Could you check a few things on this model? Use its own coordinates, in mm. A direction names the side the tool comes from. Coordinates: 2 decimals unless noted, no trailing zeros. Loops run counter-clockwise (first coordinate to the right, second up) from the corner with the lowest first, then second, coordinate; pieces in that order, holes last.
1) Imagine slicing it at B-B on z = 3. Please give me the cut outline in (x, y), plus the area to 3 significant figures.
2) If I drill on line 1 along X through (y, z) = (1, 12); line 2 along X through (y, z) = (-1.75, 9.75); line 3 along X through (y, z) = (-0.75, 12), over which ranges is the centre line in solid material (lowest first)?
3) For faces 1 (the face through (0, 0, 0)), 2 (the face through (0, 1.75, 12)), 3 (the face through (0, -2, 5)), which set-ups out of +Z, -Z, +X, -X, +Y, -Y let a thin tool reach every point of the face, with its end or its side?
4) Will these pins go through, and if not, where does the flat tip stop? P1, Ø4, axis at y = 1, z = 6, coming from the -X side; P2, Ø3, axis at x = -1.5, z = 7.5, coming from the +Y side; P3, Ø1, axis at x = -0.5, z = 11.5, coming from the +Y side.
5) Imagine slicing it at A-A on z = 10.75. Please give me the cut outline in (x, y).
```python
from build123d import *

# Parameters (mm, degrees)
SKETCH_1_R          = 2
EXTRUDE_1_DEPTH     = 10
SKETCH_2_R          = 4
EXTRUDE_2_DEPTH     = 3
CUT_EXTRUDE_1_DEPTH = 2
FILLET_1_R          = 2


with BuildPart() as part:
    # 草图1 → 凸台-拉伸1 (new body)
    with BuildSketch(Plane.XY):
        Circle(SKETCH_1_R)
    extrude(amount=EXTRUDE_1_DEPTH)

    # 草图2 → 凸台-拉伸2 (add)
    with BuildSketch(Plane.XY.offset(10)):
        Circle(SKETCH_2_R)
    extrude(amount=EXTRUDE_2_DEPTH)

    # 草图3 → 切除-拉伸1 (cut)
    with BuildSketch(Plane.XY.offset(13)):
        Polygon((2.020725942, 0), (1.010362971, 1.75), (-1.010362971, 1.75), (-2.020725942, 0), (-1.010362971, -1.75), (1.010362971, -1.75), align=None)
    extrude(amount=-CUT_EXTRUDE_1_DEPTH, mode=Mode.SUBTRACT)

    # 圆角1
    # the kernel refuses this fillet: 2 mm, written as the material it takes off along each edge
    with BuildSketch(Plane(origin=(0, 0, 13), x_dir=(1, 0, 0), z_dir=(0, -1, 0))) as fillet_1_piece_1:
        with BuildLine():
            CenterArc((4 - FILLET_1_R, -FILLET_1_R), FILLET_1_R, 0, 90)
            Line((4 - FILLET_1_R, 0), (4, 0))
            Line((4, 0), (4, -FILLET_1_R))
        make_face()
    revolve(axis=Axis((0, 0, 13), (0, 0, 1)), mode=Mode.SUBTRACT)


solid = part.part
```
Filled in:
1. outline: circle Ø4 at (0, 0)
1. area: 12.6 mm2
2. line 1: x = -3.6 to -1.44, 1.44 to 3.6
2. line 2: x = -0.97 to 0.97
2. line 3: x = -3.66 to -1.59, 1.59 to 3.66
3. face 1: -Z, +X, -X, +Y, -Y
3. face 2: +Z
3. face 3: -Z
4. P1: stops at x = -2
4. P2: stops at y = 2
4. P3: stops at y = 3.99
5. outline: circle Ø8 at (0, 0)
